The listing builds one solid part. Answer for the finished solid, in the listing's coordinates (mm). A direction names the side the tool comes from. Coordinates: 2 decimals unless noted, no trailing zeros. Order: outer loops, then holes, each group sorted by start corner. A loop starts at its lowest first (then second) coordinate and runs counter-clockwise, first axis right, second up. Notation, with made-up numbers: (25, -35) -> (31, -35) arc R24 ccw to (31, 0) -> close; hole circle Ø7 at (4, 89.25). An arc over 180 degrees is marked (long way). Return JSON: item names as keys, results as strings.
from build123d import *

# Parameters (mm, degrees)
SKETCH1_W           = 30
SKETCH1_H           = 25
BOSS_EXTRUDE1_DEPTH = 5
CHAMFER1_SIZE       = 5
BOSS_EXTRUDE4_DEPTH = 15
FILLET3_R           = 2
FILLET4_R           = 2
SKETCH12_R          = 5
BOSS_EXTRUDE5_DEPTH = 3
FILLET5_R           = 2


with BuildPart() as part:
    # Sketch1 → Boss-Extrude1 (new body)
    with BuildSketch(Plane(origin=(0, 0, 0), x_dir=(1, 0, 0), z_dir=(0, 1, 0))):
        Rectangle(SKETCH1_W, SKETCH1_H)
    extrude(amount=BOSS_EXTRUDE1_DEPTH)

    # Chamfer1
    chamfer1_edges = [part.edges().sort_by_distance(p)[0] for p in [
        (0, 5, 12.5),
        (-15, 5, 0),
        (0, 5, -12.5),
        (15, 5, 0),
    ]]
    chamfer(chamfer1_edges, length=CHAMFER1_SIZE - 0.0001)  # a hair under: the kernel refuses the full size

    # Sketch9 → Revolve1 (revolve)
    with BuildSketch(Plane.XY):
        with BuildLine():
            Line((0, 5), (0, 8))
            Line((0, 8), (3, 8))
            ThreePointArc((3, 8), (2.378679656, 6.5), (3, 5))
            Line((3, 5), (0, 5))
        make_face()
    revolve(axis=Axis((0, 5, 0), (0, 1, 0)))

    # Sketch11 → Boss-Extrude4 (add, symmetric)
    with BuildSketch(Plane(origin=(0, 0, 0), x_dir=(0, 0, -1), z_dir=(1, 0, 0))):
        Polygon((-5.616779032, 27.075000452), (6.383220968, 20.532496755), (6.383220968, 8), (-5.616779032, 8), align=None)
    extrude(amount=BOSS_EXTRUDE4_DEPTH, both=True)

    # Fillet3
    fillet3_edges = [part.edges().sort_by_distance(p)[0] for p in [
        (-15, 14.266248378, -6.383220968),
        (-15, 23.803748604, -0.383220968),
        (-15, 17.537500226, 5.616779032),
        (0, 27.075000452, 5.616779032),
        (-15, 8, -0.383220968),
        (0, 8, 5.616779032),
        (15, 14.266248378, -6.383220968),
        (15, 23.803748604, -0.383220968),
        (15, 17.537500226, 5.616779032),
        (15, 8, -0.383220968),
    ]]
    fillet(fillet3_edges, radius=FILLET3_R)

    # Fillet4
    fillet4_edges = [part.edges().sort_by_distance(p)[0] for p in [
        (10.0001, 5, 0),
        (0, 5, -7.5001),
        (-10.0001, 5, 0),
        (0, 5, 7.5001),
    ]]
    fillet(fillet4_edges, radius=FILLET4_R)

    # Sketch12 → Boss-Extrude5 (add)
    with BuildSketch(Plane.XY.offset(5.616779032)):
        with Locations(Location((0, 16.913633245, 0), (0, 0, 90))):
            Circle(SKETCH12_R)
    extrude(amount=BOSS_EXTRUDE5_DEPTH)

    # Fillet5
    fillet5_edges = [part.edges().sort_by_distance(p)[0] for p in [
        (0, 11.913633245, 8.616779032),
    ]]
    fillet(fillet5_edges, radius=FILLET5_R)


solid = part.part
1. The part is cut by section D-D on y = 9. Give the vertices of the cut face in (x, z).
Answer block:
{"outline": "(-14.73, -5.38) arc R2 ccw to (-13, -6.38) -> (13, -6.38) arc R2 ccw to (14.73, -5.38) -> (14.73, 3.62) arc R1.73 ccw to (13, 5.35) -> (-13, 5.35) arc R1.73 ccw to (-14.73, 3.62) -> close"}
2. For faces 5 (the face through (-14.43, 14.18, -5.78)), 6 (the face through (13, 2, 0)), 7 (the face through (0, 17, 8.617)), 8 (the face through (0.182, 8.601, 5.046)), determine the directions among +Z, -Z, +X, -X, +Y, -Y from which every point of the face is accessible in a straight line to the end or side of a thin tool.
Answer block:
{"face 5": "-Z, -X, +Y", "face 6": "+Z, -Z, +X", "face 7": "+Z, +X, -X, +Y", "face 8": "+Z, +X, -X"}
3. Consider line 1 (Z direction, x = -13, y = 17); line 2 (Z direction, x = 1, y = 15.5); line 3 (Y direction, x = 11.5, z = -0.5). Determine where each line is inside the solid, lowest interval first. Write a range as from..to.
Answer block:
{"line 1": "z = -6.38..5.62", "line 2": "z = -6.38..8.62", "line 3": "y = 0..3.5, 8..23.74"}
4. Each of these flat-tipped pins is pushed along its axis until it touches: pin 1 Ø6.5 at (x, y) = (0, 14.5) entering from -Z; pin 2 Ø6 at (x, z) = (7, -5) entering from +Y; pin 3 Ø5 at (x, y) = (-1, 20) entering from +Z. Where does it stop, or does it pass through?
Answer block:
{"pin 1": "stops at z = -6.38", "pin 2": "stops at y = 22.92", "pin 3": "stops at z = 8.62"}
5. Determine the mould class of faces 1 (the face through (0.182, 25.441, 4.613)), 2 (the face through (0, 0, 0)), 3 (the face through (-14.399, 16.949, 5.046)), 4 (the face through (-14.43, 8.6, -1.31)) for opening direction Y: pulls with the +Y half, pulls with the -Y half, needs draft (parallel to the pull), parting line crosses it, or undercut.
Answer block:
{"face 1": "pulls with the +Y half", "face 2": "pulls with the -Y half", "face 3": "needs draft", "face 4": "undercut"}
